Design review of the part built by this model. Coordinates are the model's own, in mm. A direction names the side the tool comes from. Coordinates: 2 decimals unless noted, no trailing zeros. Write each loop counter-clockwise with the first axis right and the second up, starting at its lowest first coordinate (ties: lowest second). Pieces come first, ordered by that corner, then holes.
Q1. Insertion check: pin 1 (1 mm diameter, centred on x = -1, y = -2.5, fed in from -Z). The pin has a flat end and moves straight along its axis. Give the tip position at first contact, or say it passes through.
Q2. Take a section at B-B (z = 0). Give the boundary of the cut face in (x, y) (3 decimals).
Q3. Machinability: for faces 4 (the flat face through (-1, 0, 1)), 5 (the flat face through (0, -6, 0)), which of the approach directions +Z, -Z, +X, -X, +Y, -Y give a long, thin tool a straight path to every point of the face, cutting with its end or side? Answer none if there is none.
Q4. For probe 1 along Y at (x, z) = (-1.05, 0.6); probe 2 along X at (y, z) = (-5.25, 0) (3 decimals); probe 3 along X at (y, z) = (1, 0.3), list the stretches that pass through material, from the lowest coordinate up.
Q5. Mouldability with a two-part tool opening along X and no side actions: class faces 1 (the flat face through (0, 0.7, 0)), 2 (the flat face through (-0.5, 1.5, 0.5)), 3 (the cylindrical face through (0.957, -2.859, 0.126)) as pulls with the +X half, pulls with the -X half, needs draft (parallel to the pull), parting line crosses it, or undercut.
Q6. Take a section at A-A (x = 0). Give the boundary of the cut face in (y, z) (3 decimals), and give its area (3 significant figures).
Q7. Take a section at C-C (y = -4.75). Give the boundary of the cut face in (x, z) (3 decimals).
```python
from build123d import *

# Parameters (mm, degrees)
SKETCH1_R                         = 1.7
BOSS_EXTRUDE1_DEPTH               = 1.5
SKETCH2_R                         = 0.965
BOSS_EXTRUDE2_DEPTH               = 6
CHAMFER1_SIZE                     = 0.2
SKETCH3_W                         = 0.5
SKETCH3_H                         = 2
CUT_EXTRUDE_THIN1_DEPTH           = 0.8
CUT_EXTRUDE_THIN1_DRAFT           = -5
SKETCH3_W_2                       = 2
SKETCH3_H_2                       = 0.5
CUT_EXTRUDE_THIN1_PROFILE_2_DEPTH = 0.8
CUT_EXTRUDE_THIN1_PROFILE_2_DRAFT = -5
FILLET1_R                         = 0.5


with BuildPart() as part:
    # Sketch1 → Boss-Extrude1 (new body)
    with BuildSketch(Plane(origin=(0, 0, 0), x_dir=(1, 0, 0), z_dir=(0, 1, 0))):
        with Locations(Location((0, 0, 0), (0, 0, 270))):
            Circle(SKETCH1_R)
    extrude(amount=BOSS_EXTRUDE1_DEPTH)

    # Sketch2 → Boss-Extrude2 (add)
    with BuildSketch(Plane.XZ):
        with Locations(Location((0, 0, 0), (0, 0, 270))):
            Circle(SKETCH2_R)
    extrude(amount=BOSS_EXTRUDE2_DEPTH)

    # Chamfer1
    chamfer1_edges = [part.edges().sort_by_distance(p)[0] for p in [
        (0, -6, 0.965),
    ]]
    chamfer(chamfer1_edges, length=CHAMFER1_SIZE)


with BuildPart() as cut_extrude_thin1_tool:
    # Sketch3 → Cut-Extrude-Thin1 (with draft: the straight prism first)
    with BuildSketch(Plane(origin=(0, 1.5, 0), x_dir=(1, 0, 0), z_dir=(0, 1, 0))):
        Rectangle(SKETCH3_W, SKETCH3_H)
    extrude(amount=-CUT_EXTRUDE_THIN1_DEPTH)
    # Cut-Extrude-Thin1: the draft: its side faces are tilted about the plane it starts from
    cut_extrude_thin1_sides = [cut_extrude_thin1_tool.faces().sort_by_distance(p)[0] for p in [
        (0.25, 1.1, 0),
        (0, 1.1, -1),
        (-0.25, 1.1, 0),
        (0, 1.1, 1),
    ]]
    draft(cut_extrude_thin1_sides, Plane(origin=(0, 1.5, 0), x_dir=(1, 0, 0), z_dir=(0, 1, 0)), CUT_EXTRUDE_THIN1_DRAFT)


with BuildPart() as part_1:
    add(part.part)

    # Cut-Extrude-Thin1: cut by cut_extrude_thin1_tool
    add(cut_extrude_thin1_tool.part, mode=Mode.SUBTRACT)


with BuildPart() as cut_extrude_thin1_profile_2_tool:
    # Sketch3 → Cut-Extrude-Thin1 profile 2 (with draft: the straight prism first)
    with BuildSketch(Plane(origin=(0, 1.5, 0), x_dir=(1, 0, 0), z_dir=(0, 1, 0))):
        Rectangle(SKETCH3_W_2, SKETCH3_H_2)
    extrude(amount=-CUT_EXTRUDE_THIN1_PROFILE_2_DEPTH)
    # Cut-Extrude-Thin1 profile 2: the draft: its side faces are tilted about the plane it starts from
    cut_extrude_thin1_profile_2_sides = [cut_extrude_thin1_profile_2_tool.faces().sort_by_distance(p)[0] for p in [
        (0, 1.1, 0.25),
        (1, 1.1, 0),
        (0, 1.1, -0.25),
        (-1, 1.1, 0),
    ]]
    draft(cut_extrude_thin1_profile_2_sides, Plane(origin=(0, 1.5, 0), x_dir=(1, 0, 0), z_dir=(0, 1, 0)), CUT_EXTRUDE_THIN1_PROFILE_2_DRAFT)


with BuildPart() as part_2:
    add(part_1.part)

    # Cut-Extrude-Thin1 profile 2: cut by cut_extrude_thin1_profile_2_tool
    add(cut_extrude_thin1_profile_2_tool.part, mode=Mode.SUBTRACT)

    # Fillet1
    fillet1_edges = [part_2.edges().sort_by_distance(p)[0] for p in [
        (0, 1.5, -1.7),
    ]]
    fillet(fillet1_edges, radius=FILLET1_R)


solid = part_2.part
```
Response:
1. pin 1: stops at z = -0.83
2. outline: (-1.7, 0) - (-0.965, 0) - (-0.965, -5.8) - (-0.765, -6) - (0.765, -6) - (0.965, -5.8) - (0.965, 0) - (1.7, 0) - (1.7, 1) arc R0.5 ccw to (1.2, 1.5) - (1, 1.5) - (0.93, 0.7) - (-0.93, 0.7) - (-1, 1.5) - (-1.2, 1.5) arc R0.5 ccw to (-1.7, 1) - close
3. face 4: -Y
3. face 5: +Z, -Z, +X, -X, -Y
4. probe 1: y = 0 to 1.5
4. probe 2: x = -0.965 to 0.965
4. probe 3: x = -1.67 to -0.21, 0.21 to 1.67
5. face 1: undercut
5. face 2: needs draft
5. face 3: parting line crosses it
6. outline: (-6, -0.765) - (-5.8, -0.965) - (0, -0.965) - (0, -1.7) - (1, -1.7) arc R0.5 ccw to (1.5, -1.2) - (1.5, -1) - (0.7, -0.93) - (0.7, 0.93) - (1.5, 1) - (1.5, 1.2) arc R0.5 ccw to (1, 1.7) - (0, 1.7) - (0, 0.965) - (-5.8, 0.965) - (-6, 0.765) - close
6. area: 15.0 mm2
7. outline: circle Ø1.93 at (0, 0)
